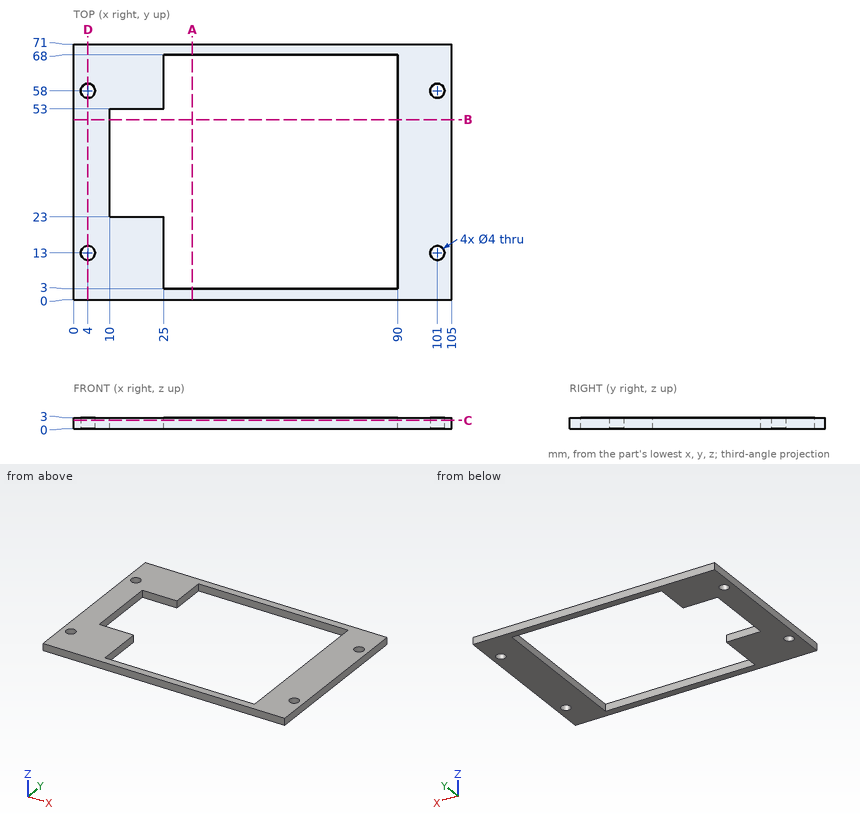
Drawing for the job (mm, zero at the part's lowest x, y, z). Round coordinates to 2 decimals unless told otherwise and drop trailing zeros. Loops run counter-clockwise (first coordinate to the right, second up) from the corner with the lowest first, then second, coordinate; pieces in that order, holes last.
1. Band-saw the part on D-D, the plane x = 4. List the corners of the cut face in (y, z).
Check values:
outline: (0, 0) - (11, 0) - (11, 3) - (0, 3) - close; (15, 0) - (56, 0) - (56, 3) - (15, 3) - close; (60, 0) - (71, 0) - (71, 3) - (60, 3) - close
2. Drop a flat-ended pin along its axis: P1, Ø3.5, axis at x = 4, y = 13, coming from the +Z side. Give the stop position or say it passes through.
Check values:
P1: passes through
3. Band-saw the part on A-A, the plane x = 33. List the corners of the cut face in (y, z).
Check values:
outline: (0, 0) - (3, 0) - (3, 3) - (0, 3) - close; (68, 0) - (71, 0) - (71, 3) - (68, 3) - close
4. Band-saw the part on C-C, the plane z = 2.3. List the corners of the cut face in (x, y), and give its area (3 significant figures).
Check values:
outline: (0, 0) - (105, 0) - (105, 71) - (0, 71) - close; hole circle Ø4 at (4, 13); hole circle Ø4 at (4, 58); hole (10, 23) - (25, 23) - (25, 3) - (90, 3) - (90, 68) - (25, 68) - (25, 53) - (10, 53) - close; hole circle Ø4 at (101, 13); hole circle Ø4 at (101, 58)
area: 2,730 mm2
5. Wall check: probe 1 along X at (y, z) = (58, 0.7); probe 2 along Y at (x, z) = (4, 1.65); probe 3 along Y at (x, z) = (83.5, 0.1). Give the ranges that are in metal, low to high.
Check values:
probe 1: x = 0 to 2, 6 to 25, 90 to 99, 103 to 105
probe 2: y = 0 to 11, 15 to 56, 60 to 71
probe 3: y = 0 to 3, 68 to 71
6. Band-saw the part on B-B, the plane y = 50. List the corners of the cut face in (x, z), and give its area (3 significant figures).
Check values:
outline: (0, 0) - (10, 0) - (10, 3) - (0, 3) - close; (90, 0) - (105, 0) - (105, 3) - (90, 3) - close
area: 75.0 mm2
